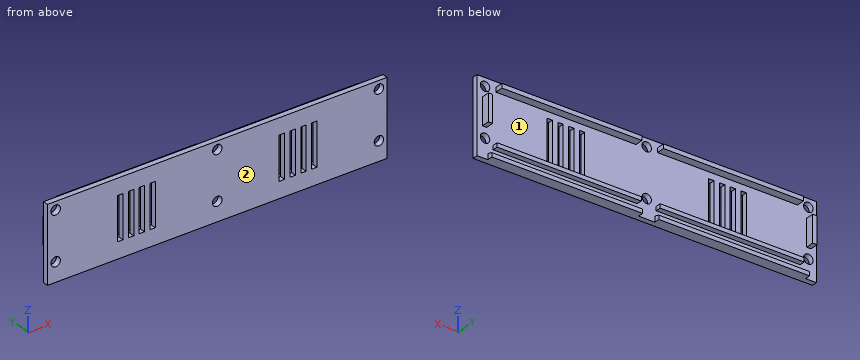
```python
from build123d import *

# Parameters (mm, degrees)
SKIZZE1_W                       = 126
SKIZZE1_H                       = 28
AUFSATZ_LINEAR_AUSTRAGEN1_DEPTH = 2
SKIZZE2_R                       = 1.75
SCHNITT_LINEAR_AUSTRAGEN1_DEPTH = 130.089116505
SKIZZE3_W                       = 2
SKIZZE3_H                       = 16
SCHNITT_LINEAR_AUSTRAGEN2_DEPTH = 130.089116505
LINEARES_MUSTER1_COUNT          = 4
LINEARES_MUSTER1_PITCH          = 4
SKIZZE4_W                       = 2
SKIZZE4_H                       = 16
SCHNITT_LINEAR_AUSTRAGEN3_DEPTH = 130.089116505
LINEARES_MUSTER2_COUNT          = 4
LINEARES_MUSTER2_PITCH          = 4
SKIZZE5_W                       = 1.6
SKIZZE5_H                       = 10
SKIZZE5_W_2                     = 52
SKIZZE5_H_2                     = 1.6
AUFSATZ_LINEAR_AUSTRAGEN2_DEPTH = 3
SKIZZE6_W                       = 53.5
SKIZZE6_H                       = 1.5
AUFSATZ_LINEAR_AUSTRAGEN3_DEPTH = 2
SKIZZE7_W                       = 56
SKIZZE7_H                       = 2.1
AUFSATZ_LINEAR_AUSTRAGEN4_DEPTH = 2
FASE1_SIZE                      = 2
FASE1_SIZE_2                    = 0.6


with BuildPart() as part:
    # Skizze1 → Aufsatz-Linear austragen1 (new body)
    with BuildSketch(Plane(origin=(0, 0, 0), x_dir=(1, 0, 0), z_dir=(0, 1, 0))):
        with Locations((63, 14)):
            Rectangle(SKIZZE1_W, SKIZZE1_H)
    extrude(amount=AUFSATZ_LINEAR_AUSTRAGEN1_DEPTH)

    # Skizze2 → Schnitt-Linear austragen1 (cut, through all)
    with BuildSketch(Plane(origin=(0, 2, 0), x_dir=(1, 0, 0), z_dir=(0, 1, 0))):
        with Locations(Location((3, 3, 0), (0, 0, 270))):
            Circle(SKIZZE2_R)
        with Locations(Location((3, 20.9, 0), (0, 0, 270))):
            Circle(SKIZZE2_R)
        with Locations(Location((63, 3, 0), (0, 0, 270))):
            Circle(SKIZZE2_R)
        with Locations(Location((63, 20.9, 0), (0, 0, 270))):
            Circle(SKIZZE2_R)
        with Locations(Location((123, 20.9, 0), (0, 0, 270))):
            Circle(SKIZZE2_R)
        with Locations(Location((123, 3, 0), (0, 0, 270))):
            Circle(SKIZZE2_R)
    extrude(amount=-SCHNITT_LINEAR_AUSTRAGEN1_DEPTH, mode=Mode.SUBTRACT)

    # Skizze3 → Schnitt-Linear austragen2 (cut, through all)
    with BuildSketch(Plane(origin=(0, 2, 0), x_dir=(1, 0, 0), z_dir=(0, 1, 0))):
        with Locations((27, 14)):
            Rectangle(SKIZZE3_W, SKIZZE3_H)
    schnitt_linear_austragen2 = extrude(amount=-SCHNITT_LINEAR_AUSTRAGEN2_DEPTH, mode=Mode.SUBTRACT)

    # Lineares Muster1: Schnitt-Linear austragen2 ×4
    with Locations(*[(i * LINEARES_MUSTER1_PITCH, 0, 0) for i in range(1, LINEARES_MUSTER1_COUNT)]):
        add(schnitt_linear_austragen2, mode=Mode.SUBTRACT)

    # Skizze4 → Schnitt-Linear austragen3 (cut, through all)
    with BuildSketch(Plane(origin=(0, 2, 0), x_dir=(1, 0, 0), z_dir=(0, 1, 0))):
        with Locations((99, 14)):
            Rectangle(SKIZZE4_W, SKIZZE4_H)
    schnitt_linear_austragen3 = extrude(amount=-SCHNITT_LINEAR_AUSTRAGEN3_DEPTH, mode=Mode.SUBTRACT)

    # Lineares Muster2: Schnitt-Linear austragen3 ×4
    with Locations(*[(-i * LINEARES_MUSTER2_PITCH, 0, 0) for i in range(1, LINEARES_MUSTER2_COUNT)]):
        add(schnitt_linear_austragen3, mode=Mode.SUBTRACT)

    # Skizze5 → Aufsatz-Linear austragen2 (add)
    with BuildSketch(Plane(origin=(0, 2, 0), x_dir=(1, 0, 0), z_dir=(0, 1, 0))):
        with Locations((2.8, 12)):
            Rectangle(SKIZZE5_W, SKIZZE5_H)
        with Locations((33, 2.8)):
            Rectangle(SKIZZE5_W_2, SKIZZE5_H_2)
        with Locations((93, 2.8)):
            Rectangle(SKIZZE5_W_2, SKIZZE5_H_2)
        with Locations((123.2, 12)):
            Rectangle(SKIZZE5_W, SKIZZE5_H)
    extrude(amount=AUFSATZ_LINEAR_AUSTRAGEN2_DEPTH)

    # Skizze6 → Aufsatz-Linear austragen3 (add)
    with BuildSketch(Plane(origin=(0, 2, 0), x_dir=(1, 0, 0), z_dir=(0, 1, 0))):
        with Locations((32.75, 23.15)):
            Rectangle(SKIZZE6_W, SKIZZE6_H)
        with Locations((93.25, 23.15)):
            Rectangle(SKIZZE6_W, SKIZZE6_H)
    extrude(amount=AUFSATZ_LINEAR_AUSTRAGEN3_DEPTH)

    # Skizze7 → Aufsatz-Linear austragen4 (add)
    with BuildSketch(Plane(origin=(0, 2, 0), x_dir=(1, 0, 0), z_dir=(0, 1, 0))):
        with Locations((32, 26.95)):
            Rectangle(SKIZZE7_W, SKIZZE7_H)
        with Locations((94, 26.95)):
            Rectangle(SKIZZE7_W, SKIZZE7_H)
    extrude(amount=AUFSATZ_LINEAR_AUSTRAGEN4_DEPTH)

    # Fase1
    # the kernel refuses this chamfer: 2, 0.6 mm, written as the material it takes off along each edge
    with BuildSketch(Plane(origin=(127.191883336, 4, -25.9), x_dir=(0, -0.9999387354199845, 0.011069119507991545), z_dir=(-1, 0, 0))) as fase1_piece_1_section:
        Polygon((FASE1_SIZE * 0.99993873542, -FASE1_SIZE * 0.011069119508), (-FASE1_SIZE_2 * 0.011069119508, -FASE1_SIZE_2 * 0.99993873542), (0, 0), align=None)
    fase1_piece_1 = extrude(amount=66.383766671, mode=Mode.PRIVATE)
    fase1_piece_1 = split(fase1_piece_1, bisect_by=Plane(origin=(94, 2, -26.081095953), z_dir=(0, 1, 0)), keep=Keep.TOP, mode=Mode.PRIVATE)
    add(fase1_piece_1, mode=Mode.SUBTRACT)
    with BuildSketch(Plane(origin=(65.191883336, 4, -25.9), x_dir=(0, -0.9999387354199845, 0.011069119507991545), z_dir=(-1, 0, 0))) as fase1_piece_2_section:
        Polygon((FASE1_SIZE * 0.99993873542, -FASE1_SIZE * 0.011069119508), (-FASE1_SIZE_2 * 0.011069119508, -FASE1_SIZE_2 * 0.99993873542), (0, 0), align=None)
    fase1_piece_2 = extrude(amount=66.383766671, mode=Mode.PRIVATE)
    fase1_piece_2 = split(fase1_piece_2, bisect_by=Plane(origin=(32, 2, -26.081095953), z_dir=(0, 1, 0)), keep=Keep.TOP, mode=Mode.PRIVATE)
    add(fase1_piece_2, mode=Mode.SUBTRACT)


solid = part.part
```
For this review, take the finished solid that the model builds, in its own axes (mm). Face numbers are marked on the shaded views. Give positions to 0.01 mm unless a question says otherwise; leave off trailing zeros. Loops run counter-clockwise (first coordinate to the right, second up) from the corner with the lowest first, then second, coordinate; pieces in that order, holes last. Notation, with made-up numbers: M -5,24 L 9,24 A16 cw 9,30 Z; hole C 39.25,-22 d8. An arc over 180 degrees is marked long. One line per item, written item: value. Start each with the question number.
Q1. Clearance check with flat-ended pins moving along their axes: pin 1 Ø0.9 at (y, z) = (3, -14) entering from -X; pin 2 Ø8 at (x, z) = (57, -23.5) entering from +Y; pin 3 Ø0.8 at (y, z) = (3.5, -3) entering from -X. State where each tip first meets the part, or that it passes through.
Q2. For L1, parallel to Z at x = 123, y = 1.25; L2, parallel to X at y = 0.5, z = -3; L3, parallel to Z at x = 82, y = 2.9, list the stretches that pass through material, from the lowest coordinate up.
Q3. Add section C-C (z = -14). Count the separate pieces of the cut face and the enclosed holes in it, and give its area (3 significant figures).
Q4. Add section A-A (x = 63). Give the boundary of the cut face in (y, z).
Q5. Add section B-B (x = 113.5). Give the boundary of the cut face in (y, z).
Q6. Draft analysis for pull direction X (two halves, no side actions). For the marked faces 1 and 2, state which applies: released by +X, released by -X, zero draft, split by the parting line, or undercut.
Reply:
1. pin 1: x = 2
1. pin 2: y = 4
1. pin 3: x = 7
2. L1: -28 to -22.65, -19.15 to -4.75, -1.25 to 0
2. L2: 0 to 1.25, 4.75 to 61.25, 64.75 to 121.25, 124.75 to 126
2. L3: -28 to -26.17, -23.9 to -22.4, -3.6 to -2
3. separate pieces: 9
3. enclosed holes: 0
3. area: 230 mm²
4. outline: M 0,-28 L 2,-28 L 2,-22.65 L 0,-22.65 Z; M 0,-19.15 L 2,-19.15 L 2,-4.75 L 0,-4.75 Z; M 0,-1.25 L 2,-1.25 L 2,0 L 0,0 Z
5. outline: M 0,-28 L 4,-28 L 4,-26.5 L 2,-25.9 L 2,-23.9 L 4,-23.9 L 4,-22.4 L 2,-22.4 L 2,-3.6 L 5,-3.6 L 5,-2 L 2,-2 L 2,0 L 0,0 Z
6. face 1: undercut
6. face 2: zero draft
